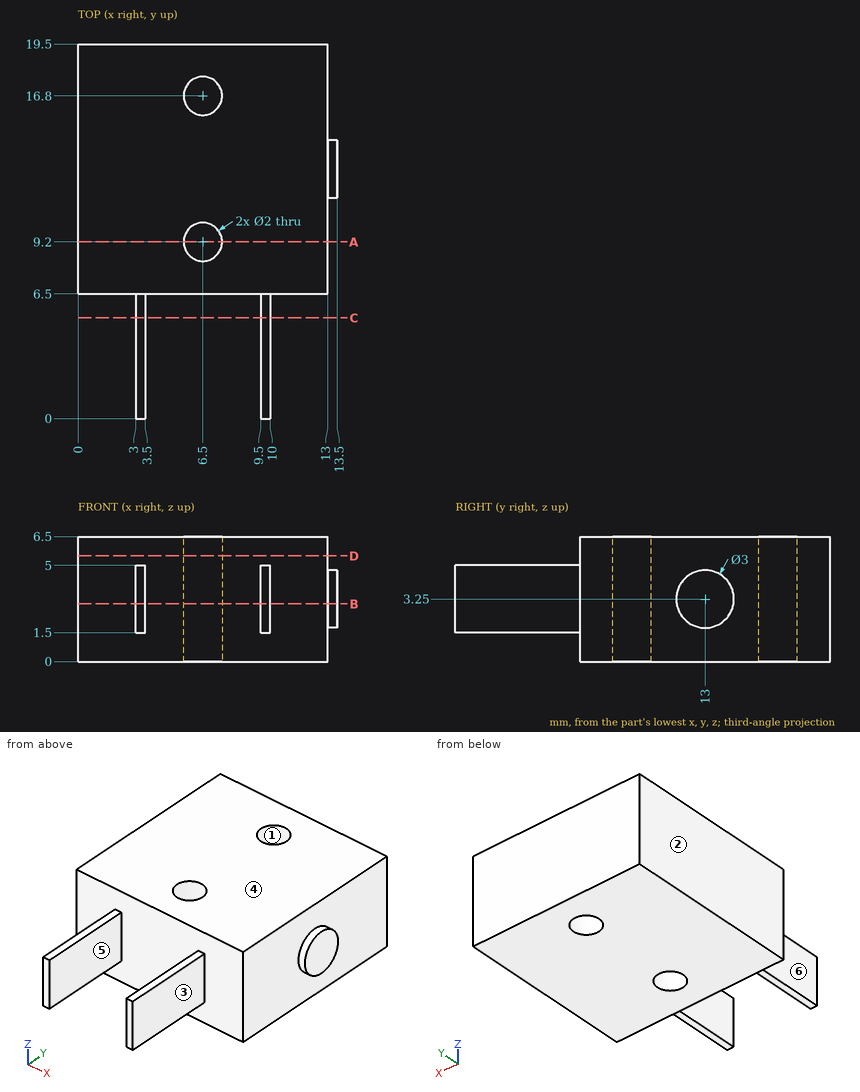
Can you work these out from the drawing? Everything is in mm from the part's minimum corner. A direction names the side the tool comes from. Give positions to 0.01 mm unless a question says otherwise; leave off trailing zeros. Loops run counter-clockwise (first coordinate to the right, second up) from the corner with the lowest first, then second, coordinate; pieces in that order, holes last. Notation, with made-up numbers: M 20,88.25 L 57,88.25 A21 ccw 57,113.25 Z; hole C 24.25,8.5 d11. An arc over 180 degrees is marked long. Put each result on its own line as item: value. Start each with the question number.
(1) I want a section at C-C on y = 5.25. Please give me the cut outline in (x, z), then the cut area to 3 significant figures.
(2) Will these pins go through, and if not, where does the flat tip stop? pin 1 Ø1 at (y, z) = (3, 4) entering from +X; pin 2 Ø1.8 at (y, z) = (4, 4) entering from -X; pin 3 Ø2 at (y, z) = (10, 4.5) entering from +X.
(3) I need wall thicknesses on line 1 along Y through (x, z) = (6.5, 5); line 2 along X through (y, z) = (10.5, 4.5); line 3 along Y through (x, z) = (4.25, 3.5). Which ranges of each line are inside material? Lowest first, please. Write a range as [from, to].
(4) I want a section at D-D on z = 5.5. Please give me the cut outline in (x, y).
(5) If we mould it in two halves opening along X, with no side actions, what happens to the marked faces 1, 2 and 3? For each: +X half, -X half, draft (parallel to the pull), parting line (faces both ways), or undercut.
(6) For the marked faces 4, 5 and 6, which set-ups out of +Z, -Z, +X, -X, +Y, -Y let a thin tool reach every point of the face, with its end or its side?
(7) I want a section at B-B on z = 3. Please give me the cut outline in (x, y), then the cut area to 3 significant figures.
(8) I want a section at A-A on y = 9.2. Please give me the cut outline in (x, z).
Answer block:
1. outline: M 3,1.5 L 3.5,1.5 L 3.5,5 L 3,5 Z; M 9.5,1.5 L 10,1.5 L 10,5 L 9.5,5 Z
1. area: 3.50 mm^2
2. pin 1: x = 10
2. pin 2: x = 3
2. pin 3: x = 13
3. line 1: [6.5, 8.2], [10.2, 15.8], [17.8, 19.5]
3. line 2: [0, 13]
3. line 3: [6.5, 19.5]
4. outline: M 0,6.5 L 13,6.5 L 13,19.5 L 0,19.5 Z; hole C 6.5,9.2 d2; hole C 6.5,16.8 d2
5. face 1: undercut
5. face 2: -X half
5. face 3: +X half
6. face 4: +Z, +X, -X, +Y, -Y
6. face 5: +Z, -Z, -Y
6. face 6: +Z, -Z, -X, -Y
7. outline: M 0,6.5 L 3,6.5 L 3,0 L 3.5,0 L 3.5,6.5 L 9.5,6.5 L 9.5,0 L 10,0 L 10,6.5 L 13,6.5 L 13,11.52 L 13.5,11.52 L 13.5,14.48 L 13,14.48 L 13,19.5 L 0,19.5 Z; hole C 6.5,9.2 d2; hole C 6.5,16.8 d2
7. area: 171 mm^2
8. outline: M 0,0 L 5.5,0 L 5.5,6.5 L 0,6.5 Z; M 7.5,0 L 13,0 L 13,6.5 L 7.5,6.5 Z
